from build123d import *

# Parameters (mm, degrees)
BOSS_EXTRUDE1_DEPTH = 15
SKETCH2_R           = 2.625
CUT_EXTRUDE1_DEPTH  = 10
FILLET3_R           = 5
FILLET5_R           = 1
FILLET6_R           = 1
SKETCH3_R           = 1.5
CUT_EXTRUDE4_DEPTH  = 58


with BuildPart() as part:
    # Sketch1 → Boss-Extrude1 (new body)
    with BuildSketch(Plane.XY):
        with BuildLine():
            ThreePointArc((-5, -15.142135624), (0, 14), (5, -15.142135624))
            Line((5, -15.142135624), (5, -35.142135624))
            Line((5, -35.142135624), (9, -35.142135624))
            Line((9, -35.142135624), (9, -17.860571099))
            ThreePointArc((9, -17.860571099), (19.980623019, -0.880172578), (10.535653753, 17))
            Line((10.535653753, 17), (30, 17))
            Line((30, 17), (30, 35.5))
            Line((30, 35.5), (26, 35.5))
            Line((26, 35.5), (26, 21))
            Line((26, 21), (-26, 21))
            Line((-26, 21), (-26, 35.5))
            Line((-26, 35.5), (-30, 35.5))
            Line((-30, 35.5), (-30, 17))
            Line((-30, 17), (-10.535653753, 17))
            ThreePointArc((-10.535653753, 17), (-19.980623019, -0.880172578), (-9, -17.860571099))
            Line((-9, -17.860571099), (-9, -35.142135624))
            Line((-9, -35.142135624), (-5, -35.142135624))
            Line((-5, -35.142135624), (-5, -15.142135624))
        make_face()
    extrude(amount=BOSS_EXTRUDE1_DEPTH)

    # Sketch2 → Cut-Extrude1 (cut)
    with BuildSketch(Plane(origin=(9, 0, 0), x_dir=(0, 0, -1), z_dir=(1, 0, 0))):
        with Locations(Location((-7.5, -27.860571099, 0), (0, 0, 90))):
            Circle(SKETCH2_R)
    extrude(amount=-CUT_EXTRUDE1_DEPTH, mode=Mode.SUBTRACT)

    # Fillet3
    fillet3_edges = [part.edges().sort_by_distance(p)[0] for p in [
        (9, -17.860571099, 7.5),
        (-9, -17.860571099, 7.5),
    ]]
    fillet(fillet3_edges, radius=FILLET3_R)

    # Fillet5
    fillet5_edges = [part.edges().sort_by_distance(p)[0] for p in [
        (10.535653753, 17, 7.5),
        (-10.535653753, 17, 7.5),
    ]]
    fillet(fillet5_edges, radius=FILLET5_R)

    # Fillet6
    fillet6_edges = [part.edges().sort_by_distance(p)[0] for p in [
        (26, 21, 7.5),
        (-26, 21, 7.5),
        (-30, 17, 7.5),
        (30, 17, 7.5),
    ]]
    fillet(fillet6_edges, radius=FILLET6_R)

    # Sketch3 → Cut-Extrude4 (cut)
    with BuildSketch(Plane(origin=(30, 0, 0), x_dir=(0, 0, -1), z_dir=(1, 0, 0))):
        with Locations((-7.5, 15.238095238)):
            Circle(SKETCH3_R)
    extrude(amount=-CUT_EXTRUDE4_DEPTH, mode=Mode.SUBTRACT)


solid = part.part
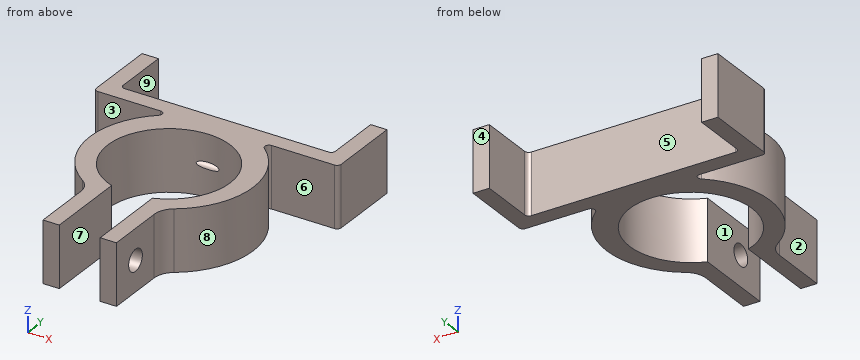
Source: CAD feature listing. Evaluate the final solid. Frame: model axes, mm. Face numbers are marked on the shaded views. A direction names the side the tool comes from. Round coordinates to 2 decimals unless told otherwise and drop trailing zeros. Order: outer loops, then holes, each group sorted by start corner. A loop starts at its lowest first (then second) coordinate and runs counter-clockwise, first axis right, second up. Notation, with made-up numbers: (83.25, 79) - (115.25, 79) arc R14 ccw to (115.25, 97) - close; hole circle Ø9 at (11, 60.25). An arc over 180 degrees is marked (long way). Use a Markdown table: item, result. Add a question column.
1. Section query C-C (z = 7.5). Give the number of separate pieces and of enclosed holes in the cut face, then the cut area to 3 significant figures.
2. Section query D-D (z = 11). Return the cut outline in (x, y).
3. Line query: probe 1 along Z at (x, y) = (0.5, 15); probe 2 along X at (y, z) = (29.5, 10.5); probe 3 along X at (y, z) = (-24.5, 8). Output: solid intervals per line, ascending.
4. Section query B-B (x = -7.5). Return the cut outline in (y, z), then the cut area to 3 significant figures.
5. Set-up query: the marked faces 1, 2, 3, 4 and 5. Return all of +Z, -Z, +X, -X, +Y, -Y with unobstructed straight access to the full face (end or side cutting, diameter ignored); none if empty.
6. Mould query, pull axis X, two halves, no side actions, for the marked faces 6, 7, 8 and 9. Classes: +X half, -X half, draft (parallel to the pull), parting line (faces both ways), or undercut.
7. First-contact query: pin 1 (6 mm diameter, centred on x = 4, z = 8.5, fed in from -Y); pin 2 (8 mm diameter, centred on y = -27, z = 8, fed in from -X); pin 3 (4.5 mm diameter, centred on y = -29, z = 8, fed in from +X); pin 4 (6 mm diameter, centred on x = -17, z = 11, fed in from -Y). Flat tips, straight axial feed; report the tip coordinate or a pass-through.
8. Section query A-A (y = -23). Return the cut outline in (x, z), then the cut area to 3 significant figures.
Derived:
| question | item | result |
|---|---|---|
| 1 | separate pieces | 4 |
| 1 | enclosed holes | 0 |
| 1 | area | 860 mm2 |
| 2 | outline | (-30, 18) arc R1 ccw to (-29, 17) - (-13.6, 17) arc R1 cw to (-12.95, 15.24) arc R20 ccw to (-11.2, -16.57) arc R5 cw to (-9, -20.71) - (-9, -35.14) - (-5, -35.14) - (-5, -15.14) arc R15 cw (long way) to (5, -15.14) - (5, -35.14) - (9, -35.14) - (9, -20.71) arc R5 cw to (11.2, -16.57) arc R20 ccw to (12.95, 15.24) arc R1 cw to (13.6, 17) - (29, 17) arc R1 ccw to (30, 18) - (30, 35.5) - (26, 35.5) - (26, 22) arc R1 cw to (25, 21) - (-25, 21) arc R1 cw to (-26, 22) - (-26, 35.5) - (-30, 35.5) - close |
| 3 | probe 1 | 0 to 6.02, 8.98 to 15 |
| 3 | probe 2 | -30 to -26, 26 to 30 |
| 3 | probe 3 | -9 to -5, 5 to 9 |
| 4 | outline | (-35.14, 0) - (-13.99, 0) - (-13.99, 15) - (-35.14, 15) - close; (11.99, 0) - (21, 0) - (21, 15) - (11.99, 15) - close; hole circle Ø3 at (15.24, 7.5) |
| 4 | area | 445 mm2 |
| 5 | face 1 | +Z, -Z, -Y |
| 5 | face 2 | +Z, -Z, -X, -Y |
| 5 | face 3 | +Z, -Z, -X |
| 5 | face 4 | +Z, -Z, +X, -X, +Y |
| 5 | face 5 | +Z, -Z, +Y |
| 6 | face 6 | draft |
| 6 | face 7 | undercut |
| 6 | face 8 | +X half |
| 6 | face 9 | undercut |
| 7 | pin 1 | y = -35.14 |
| 7 | pin 2 | x = -9 |
| 7 | pin 3 | x = 9 |
| 7 | pin 4 | y = -14.28 |
| 8 | outline | (-9, 0) - (-5, 0) - (-5, 15) - (-9, 15) - close; (5, 0) - (9, 0) - (9, 15) - (5, 15) - close |
| 8 | area | 120 mm2 |
